Could you check a few things on this model? Use its own coordinates, in mm. Face numbers are marked on the shaded views. Give positions to 0.01 mm unless a question says otherwise; leave off trailing zeros. Write each loop counter-clockwise with the first axis right and the second up, starting at its lowest first coordinate (ties: lowest second). Pieces come first, ordered by that corner, then holes. Notation, with made-up numbers: (66.5, 62.5) - (88.5, 62.5) arc R16 ccw to (88.5, 88.5) - close; hole circle Ø2 at (84, 68). An arc over 180 degrees is marked (long way). Use one line per item in the form item = value.
```python
from build123d import *

# Parameters (mm, degrees)
EXTRUDE1_DEPTH     = 158.75
SKETCH2_W          = 18.9992
SKETCH2_H          = 9.56647298
CUT_EXTRUDE1_DEPTH = 158.75
SKETCH3_R          = 4.15925
CUT_EXTRUDE2_DEPTH = 158.75
SKETCH4_R          = 6.25475
CUT_EXTRUDE3_DEPTH = 8.8392
EXTRUDE2_REACH     = 172.226


with BuildPart() as part:
    # Sketch1 → Extrude1 (new body)
    with BuildSketch(Plane.XY):
        Polygon((-16.638134778, 6.4008), (-16.638134778, 0), (52.449865222, 0), (52.449865222, 6.4008), (46.480865222, 6.4008), (46.480865222, 18.9484), (52.449865222, 18.9484), (52.449865222, 32.004), (-16.638134778, 32.004), (-16.638134778, 18.9484), (-10.669134778, 18.9484), (-10.669134778, 6.4008), align=None)
    extrude(amount=EXTRUDE1_DEPTH)

    # Sketch2 → Cut-Extrude1 (cut)
    with BuildSketch(Plane.ZY.offset(16.638134778)):
        with Locations((12.0396, 34.24723649)):
            Rectangle(SKETCH2_W, SKETCH2_H)
        with Locations((146.7104, 34.24723649)):
            Rectangle(SKETCH2_W, SKETCH2_H)
    extrude(amount=-CUT_EXTRUDE1_DEPTH, mode=Mode.SUBTRACT)

    # Sketch3 → Cut-Extrude2 (cut)
    with BuildSketch(Plane(origin=(0, 29.464, 0), x_dir=(-1, 0, 0), z_dir=(0, 1, 0))):
        with Locations(Location((3.684134778, 12.09675, 0), (0, 0, 90))):
            Circle(SKETCH3_R)
        with Locations(Location((-39.495865222, 12.09675, 0), (0, 0, 90))):
            Circle(SKETCH3_R)
        with Locations(Location((-39.495865222, 146.65325, 0), (0, 0, 90))):
            Circle(SKETCH3_R)
        with Locations(Location((3.684134778, 146.65325, 0), (0, 0, 90))):
            Circle(SKETCH3_R)
    extrude(amount=-CUT_EXTRUDE2_DEPTH, mode=Mode.SUBTRACT)

    # Sketch4 → Cut-Extrude3 (cut)
    with BuildSketch(Plane.XZ):
        with Locations(Location((-3.684134778, 146.65325, 0), (0, 0, 270))):
            Circle(SKETCH4_R)
        with Locations(Location((39.495865222, 146.65325, 0), (0, 0, 270))):
            Circle(SKETCH4_R)
        with Locations(Location((39.495865222, 12.09675, 0), (0, 0, 90))):
            Circle(SKETCH4_R)
        with Locations(Location((-3.684134778, 12.09675, 0), (0, 0, 90))):
            Circle(SKETCH4_R)
    extrude(amount=-CUT_EXTRUDE3_DEPTH, mode=Mode.SUBTRACT)

    # Sketch5 → Extrude2 (cut, up to next)
    with BuildSketch(Plane.XY, mode=Mode.PRIVATE) as extrude2_sk1:
        Polygon((8.253865222, 18.669), (5.586865222, 18.669), (5.586865222, 8.763), (30.224865222, 8.763), (30.224865222, 18.669), (27.557865222, 18.669), (27.557865222, 32.004), (8.253865222, 32.004), align=None)
    extrude2_tool1 = extrude(extrude2_sk1.sketch, amount=EXTRUDE2_REACH, mode=Mode.PRIVATE) & part.part
    add(extrude2_tool1.solids().sort_by_distance((17.905865, 19.680981, 0))[0], mode=Mode.SUBTRACT)


solid = part.part
```
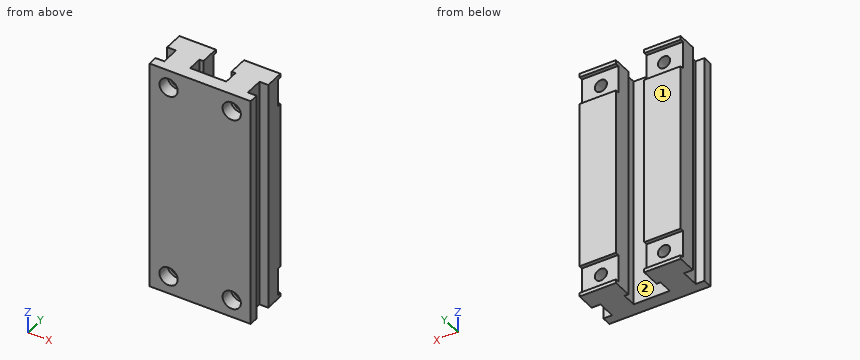
1. If we mould it in two halves opening along X, with no side actions, what happens to the marked faces 1 and 2? For each: pulls with the +X half, pulls with the -X half, needs draft (parallel to the pull), parting line crosses it, or undercut.
Response values:
face_1 = needs draft
face_2 = undercut
2. Imagine slicing it at C-C, the plane z = 48. List the corners of the cut face in (x, y) for me, and give its area (3 significant figures).
Response values:
outline = (-16.64, 0) - (52.45, 0) - (52.45, 6.4) - (46.48, 6.4) - (46.48, 18.95) - (52.45, 18.95) - (52.45, 32) - (27.56, 32) - (27.56, 18.67) - (30.22, 18.67) - (30.22, 8.76) - (5.59, 8.76) - (5.59, 18.67) - (8.25, 18.67) - (8.25, 32) - (-16.64, 32) - (-16.64, 18.95) - (-10.67, 18.95) - (-10.67, 6.4) - (-16.64, 6.4) - close
area = 1,560 mm²
3. Imagine slicing it at D-D, the plane y = 3. List the corners of the cut face in (x, z) for me, and give its area (3 significant figures).
Response values:
outline = (-16.64, 0) - (52.45, 0) - (52.45, 158.75) - (-16.64, 158.75) - close; hole circle Ø12.51 at (-3.68, 12.1); hole circle Ø12.51 at (-3.68, 146.65); hole circle Ø12.51 at (39.5, 12.1); hole circle Ø12.51 at (39.5, 146.65)
area = 10,500 mm²
4. If I drill on line 1 (X direction, y = 10.5, z = 143); line 2 (Y direction, x = 29, z = 39.5); line 3 (Y direction, x = -13, z = 122.5), over which ranges is the centre line in solid material (lowest first)? Write a range as from..to.
Response values:
line_1 = -10.67..-5.67, -1.7..5.59, 30.22..37.51, 41.48..46.48
line_2 = 0..8.76, 18.67..32
line_3 = 0..6.4, 18.95..32
5. Imagine slicing it at A-A, the plane y = 26.5. List the corners of the cut face in (x, z) for me, and give its area (3 significant figures).
Response values:
outline = (-16.64, 0) - (8.25, 0) - (8.25, 158.75) - (-16.64, 158.75) - close; (27.56, 0) - (52.45, 0) - (52.45, 158.75) - (27.56, 158.75) - close; hole circle Ø8.32 at (-3.68, 12.1); hole circle Ø8.32 at (-3.68, 146.65); hole circle Ø8.32 at (39.5, 12.1); hole circle Ø8.32 at (39.5, 146.65)
area = 7,690 mm²
6. Imagine slicing it at B-B, the plane x = -6. List the corners of the cut face in (y, z) for me.
Response values:
outline = (0, 0) - (32, 0) - (32, 2.54) - (29.46, 2.54) - (29.46, 8.64) - (8.84, 8.64) - (8.84, 6.29) - (0, 6.29) - close; (0, 17.91) - (8.84, 17.91) - (8.84, 15.55) - (29.46, 15.55) - (29.46, 21.54) - (32, 21.54) - (32, 137.21) - (29.46, 137.21) - (29.46, 143.2) - (8.84, 143.2) - (8.84, 140.84) - (0, 140.84) - close; (0, 152.46) - (8.84, 152.46) - (8.84, 150.11) - (29.46, 150.11) - (29.46, 156.21) - (32, 156.21) - (32, 158.75) - (0, 158.75) - close
7. For pin 1 (11.5 mm diameter, centred on x = 39.5, z = 12.1, fed in from -Y); pin 2 (5 mm diameter, centred on x = 2, z = 132, fed in from -Y); pin 3 (7.5 mm diameter, centred on x = 23, z = 58.5, fed in from +Y); pin 4 (5.5 mm diameter, centred on x = -4, z = 144, fed in from +Y), each with a flat end and sliding along its axis, tell me the tip position at first contact or that it passes through.
Response values:
pin_1 = 8.84
pin_2 = 0
pin_3 = 8.76
pin_4 = 29.46
